For this review, take the finished solid that the model builds, in its own axes (mm). A direction names the side the tool comes from. Give positions to 0.01 mm unless a question says otherwise; leave off trailing zeros. Loops run counter-clockwise (first coordinate to the right, second up) from the corner with the lowest first, then second, coordinate; pieces in that order, holes last. Notation, with made-up numbers: (3, 60.5) - (15, 60.5) arc R26 ccw to (15, 99.5) - close; hole circle Ø3 at (69, 64.25). An arc over 180 degrees is marked (long way). Put each result on its own line as item: value. Start each with the question number.
from build123d import *

# Parameters (mm, degrees)
SKETCH1_W           = 30
SKETCH1_H           = 16
BOSS_EXTRUDE1_DEPTH = 20
CUT_EXTRUDE1_DEPTH  = 20
SKETCH3_W           = 6
SKETCH3_H           = 10
BOSS_EXTRUDE2_DEPTH = 5
SKETCH9_R           = 1.6
CUT_EXTRUDE3_DEPTH  = 6.5
SKETCH11_W          = 10
SKETCH11_H          = 8
BOSS_EXTRUDE4_DEPTH = 40
CHAMFER2_SIZE2      = 10
CHAMFER2_SIZE       = 2
FILLET1_R           = 1
CUT_EXTRUDE4_DEPTH  = 8
SKETCH13_W          = 2
SKETCH13_H          = 8
BOSS_EXTRUDE5_DEPTH = 10
LPATTERN1_COUNT     = 8
LPATTERN1_PITCH     = 5.75
FILLET2_R           = 1
FILLET3_R           = 1
SKETCH14_W          = 2
SKETCH14_H          = 8
CUT_EXTRUDE5_DEPTH  = 5


# Some blends are built 0.0001 mm under size
with BuildPart() as part:
    # Sketch1 → Boss-Extrude1 (new body)
    with BuildSketch(Plane.XY):
        with Locations((15, -8)):
            Rectangle(SKETCH1_W, SKETCH1_H)
    extrude(amount=BOSS_EXTRUDE1_DEPTH)

    # Sketch2 → Cut-Extrude1 (cut)
    with BuildSketch(Plane.XY.offset(20)):
        Polygon((22, -6.5), (22, -8), (30, -8), (30, -16), (6, -16), (6, -6.5), align=None)
    extrude(amount=-CUT_EXTRUDE1_DEPTH, mode=Mode.SUBTRACT)

    # Sketch3 → Boss-Extrude2 (add)
    with BuildSketch(Plane.XZ.offset(16)):
        with Locations((3, 10)):
            Rectangle(SKETCH3_W, SKETCH3_H)
    extrude(amount=BOSS_EXTRUDE2_DEPTH)

    # Sketch9 → Cut-Extrude3 (cut)
    with BuildSketch(Plane.XZ.offset(6.5)):
        with Locations(Location((18, 15, 0), (0, 0, 270))):
            Circle(SKETCH9_R)
        with Locations(Location((18, 5, 0), (0, 0, 270))):
            Circle(SKETCH9_R)
    extrude(amount=-CUT_EXTRUDE3_DEPTH, mode=Mode.SUBTRACT)

    # Sketch11 → Boss-Extrude4 (add)
    with BuildSketch(Plane.XY.offset(15)):
        with Locations((3, -17)):
            Rectangle(SKETCH11_W, SKETCH11_H)
    extrude(amount=BOSS_EXTRUDE4_DEPTH)

    # Chamfer2
    chamfer2_edges = [part.edges().sort_by_distance(p)[0] for p in [
        (0, -17, 15),
    ]]
    chamfer2_side = [part.faces().sort_by_distance(p)[0] for p in [
        (-0.04, -17, 15),
    ]]
    chamfer(chamfer2_edges, length=CHAMFER2_SIZE - 0.0001, length2=CHAMFER2_SIZE2 - 0.0001, reference=chamfer2_side[0])  # a hair under: the kernel refuses the full size

    # Fillet1
    fillet1_edges = [part.edges().sort_by_distance(p)[0] for p in [
        (3, -13, 20),
    ]]
    fillet(fillet1_edges, radius=FILLET1_R)

    # Sketch12 → Cut-Extrude4 (cut)
    with BuildSketch(Plane.XZ.offset(21)):
        Polygon((7, 55), (4.75, 54.25), (2, 53.25), (2, 51.75), (4.75, 50.75), (7, 50), (7, 49.25), (8, 49.25), (8, 55), align=None)
    cut_extrude4 = extrude(amount=-CUT_EXTRUDE4_DEPTH, mode=Mode.SUBTRACT)

    # Sketch13 → Boss-Extrude5 (add)
    with BuildSketch(Plane(origin=(0, 0, 15), x_dir=(-1, 0, 0), z_dir=(0, 0, -1))):
        with Locations((-7, -17)):
            Rectangle(SKETCH13_W, SKETCH13_H)
    extrude(amount=BOSS_EXTRUDE5_DEPTH)

    # LPattern1: Cut-Extrude4 ×8
    with Locations(*[(0, 0, -i * LPATTERN1_PITCH) for i in range(1, LPATTERN1_COUNT)]):
        add(cut_extrude4, mode=Mode.SUBTRACT)

    # Fillet2
    # the kernel refuses this fillet: 1 mm, written as the material it adds along each edge
    with BuildSketch(Plane(origin=(2, -21, 51.75), x_dir=(0.9397934234884382, 0, -0.3417430630867014), z_dir=(0, 1, 0)), Plane(origin=(2, -21, 53.25), x_dir=(0, 0, -1), z_dir=(0, 1, 0)), Plane(origin=(2, -21, 46), x_dir=(0.9397934234884356, 0, -0.34174306308670804), z_dir=(0, 1, 0)), Plane(origin=(2, -21, 47.5), x_dir=(0, 0, -1), z_dir=(0, 1, 0)), Plane(origin=(2, -21, 40.25), x_dir=(0.9397934234884383, 0, -0.3417430630867007), z_dir=(0, 1, 0)), Plane(origin=(2, -21, 41.75), x_dir=(0, 0, -1), z_dir=(0, 1, 0)), Plane(origin=(2, -21, 28.75), x_dir=(0.939793423488437, 0, -0.3417430630867048), z_dir=(0, 1, 0)), Plane(origin=(2, -21, 30.25), x_dir=(0, 0, -1), z_dir=(0, 1, 0)), Plane(origin=(2, -21, 34.5), x_dir=(0.9397934234884383, 0, -0.3417430630867007), z_dir=(0, 1, 0)), Plane(origin=(2, -21, 36), x_dir=(0, 0, -1), z_dir=(0, 1, 0)), Plane(origin=(2, -21, 24.5), x_dir=(0, 0, -1), z_dir=(0, 1, 0)), Plane(origin=(2, -21, 23), x_dir=(0.939793423488437, 0, -0.3417430630867048), z_dir=(0, 1, 0))) as fillet2_piece_1:
        with BuildLine():
            CenterArc((FILLET2_R * 0.700427264611, -FILLET2_R), FILLET2_R, 90, 70.016893478)
            Line((-FILLET2_R * 0.239366158878, -FILLET2_R * 0.658256936913), (0, 0))
            Line((0, 0), (FILLET2_R * 0.700427264611, 0))
        make_face()
    extrude(amount=8)
    with BuildSketch(Plane(origin=(2, -21, 11.5), x_dir=(0.939793423488437, 0, -0.3417430630867044), z_dir=(0, 1, 0)), Plane(origin=(2, -21, 13), x_dir=(0, 0, -1), z_dir=(0, 1, 0)), Plane(origin=(2, -21, 17.25), x_dir=(0.939793423488437, 0, -0.3417430630867048), z_dir=(0, 1, 0))) as fillet2_piece_2:
        with BuildLine():
            CenterArc((FILLET2_R * 0.700427264611, -FILLET2_R), FILLET2_R, 90, 70.016893478)
            Line((-FILLET2_R * 0.239366158878, -FILLET2_R * 0.658256936913), (0, 0))
            Line((0, 0), (FILLET2_R * 0.700427264611, 0))
        make_face()
    extrude(amount=9.751068162)
    with BuildSketch(Plane(origin=(2, -21, 18.75), x_dir=(0.9397934234884369, 0, 0.34174306308670505), z_dir=(0, 1, 0))) as fillet2_piece_3:
        with BuildLine():
            CenterArc((FILLET2_R * 0.700427264611, FILLET2_R), FILLET2_R, 199.983106522, 70.016893478)
            Line((-FILLET2_R * 0.239366158878, FILLET2_R * 0.658256936913), (0, 0))
            Line((0, 0), (FILLET2_R * 0.700427264611, 0))
        make_face()
    extrude(amount=9.751068162)
    # the kernel refuses this fillet: 1 mm, written as the material it takes off along each edge
    with BuildSketch(Plane(origin=(7, -22.80189805, 26.25), x_dir=(-0.9486832980505139, 0, -0.31622776601683794), z_dir=(0, 1, 0)), Plane(origin=(7, -22.80189805, 27), x_dir=(0, 0, -1), z_dir=(0, 1, 0)), Plane(origin=(7, -22.80189805, 32), x_dir=(-0.9486832980505122, 0, -0.31622776601684277), z_dir=(0, 1, 0)), Plane(origin=(7, -22.80189805, 32.75), x_dir=(0, 0, -1), z_dir=(0, 1, 0)), Plane(origin=(7, -22.80189805, 37.75), x_dir=(-0.9486832980505133, 0, -0.31622776601683944), z_dir=(0, 1, 0)), Plane(origin=(7, -22.80189805, 38.5), x_dir=(0, 0, -1), z_dir=(0, 1, 0)), Plane(origin=(7, -22.80189805, 43.5), x_dir=(-0.9486832980505137, 0, -0.31622776601683833), z_dir=(0, 1, 0)), Plane(origin=(7, -22.80189805, 44.25), x_dir=(0, 0, -1), z_dir=(0, 1, 0)), Plane(origin=(7, -22.80189805, 49.25), x_dir=(-0.9486832980505137, 0, -0.31622776601683833), z_dir=(0, 1, 0)), Plane(origin=(7, -22.80189805, 50), x_dir=(0, 0, -1), z_dir=(0, 1, 0)), Plane(origin=(7, -22.80189805, 14.75), x_dir=(-0.9486832980505139, 0, -0.31622776601683794), z_dir=(0, 1, 0)), Plane(origin=(7, -22.80189805, 15.5), x_dir=(0, 0, -1), z_dir=(0, 1, 0)), Plane(origin=(7, -22.80189805, 20.5), x_dir=(-0.9486832980505137, 0, -0.3162277660168387), z_dir=(0, 1, 0)), Plane(origin=(7, -22.80189805, 21.25), x_dir=(0, 0, -1), z_dir=(0, 1, 0))) as fillet2_2_piece_1:
        with BuildLine():
            CenterArc((FILLET2_R * 0.720759220056, FILLET2_R), FILLET2_R, 198.434948823, 71.565051177)
            Line((-FILLET2_R * 0.227924077994, FILLET2_R * 0.683772233983), (0, 0))
            Line((0, 0), (FILLET2_R * 0.720759220056, 0))
        make_face()
    extrude(amount=11.6037961, mode=Mode.SUBTRACT)

    # Fillet3
    # the kernel refuses this fillet: 1 mm, written as the material it takes off along each edge
    with BuildSketch(Plane(origin=(7, -29.045614591, 55), x_dir=(-1, 0, 0), z_dir=(0, 1, 0))) as fillet3_piece_1:
        with BuildLine():
            CenterArc((3.218245837, -1), FILLET3_R, 90, 75.522487814)
            Line((2.25, -0.75), (2.230635083, -0.745))
            ThreePointArc((2.230635083, -0.745), (1.118675445, -0.393973666), (-0.006324555, -0.018973666))
            Line((-0.006324555, -0.018973666), (0, 0.02))
            Line((0, 0.02), (3.218245837, 0.02))
            Line((3.218245837, 0.02), (3.218245837, 0))
        make_face()
    extrude(amount=24.091229183, mode=Mode.SUBTRACT)

    # Sketch14 → Cut-Extrude5 (cut)
    with BuildSketch(Plane(origin=(0, 0, 5), x_dir=(-1, 0, 0), z_dir=(0, 0, -1))):
        with Locations((-7, -17)):
            Rectangle(SKETCH14_W, SKETCH14_H)
    extrude(amount=-CUT_EXTRUDE5_DEPTH, mode=Mode.SUBTRACT)


solid = part.part
1) Take a section at A-A on x = 18. State the section outline as (y, z) points.
2) Mouldability with a two-part tool opening along Z and no side actions: class faces 1 (the flat face through (5.5, -17.1, 50.5)), 2 (the flat face through (5.5, -17.1, 16)), 3 (the flat face through (14, -6.5, 10)) as released by +Z, released by -Z, zero draft, split by the parting line, or undercut.
3) Insertion check: P1, Ø0.8, axis at y = -7.5, z = 15, coming from the -X side; P2, Ø1, axis at x = 6, y = -9.5, coming from the +Z side; P3, Ø2.5, axis at x = 18, z = 5, coming from the -Y side; P4, Ø2.5, axis at x = 26.5, z = 14.5, coming from the -Y side. Each pin has a flat end and moves straight along its axis. Give the tip position at first contact, or say it passes through.
4) Take a section at C-C on z = 4. State the section outline as (x, y) points, and give its area (3 significant figures).
5) Take a section at B-B on y = -5. State the section outline as (x, z) points.
6) Wall thickness on probe 1 along X at (y, z) = (-5, 5); probe 2 along Z at (x, y) = (11, -0.75); probe 3 along X at (y, z) = (-9.5, 17.5): over which ranges is each line inside the solid? List them lowest first.
7) Machinability: for faces 4 (the flat face through (5.522, -17.056, 44.743)), 5 (the flat face through (22, -7, 10)), 6 (the flat face through (3, -18, 5)), 7 (the flat face through (3.719, -17.056, 13.625)), 8 (the flat face through (-2, -17, 35)), which of the approach directions +Z, -Z, +X, -X, +Y, -Y give a long, thin tool a straight path to every point of the face, cutting with its end or side? Answer none if there is none.
8) Take a section at D-D on y = -9.25. State the section outline as (x, z) points, and give its area (3 significant figures).
Answers follow:
1. outline: (-6.5, 0) - (0, 0) - (0, 3.4) - (-6.5, 3.4) - close; (-6.5, 6.6) - (0, 6.6) - (0, 13.4) - (-6.5, 13.4) - close; (-6.5, 16.6) - (0, 16.6) - (0, 20) - (-6.5, 20) - close
2. face 1: released by +Z
2. face 2: undercut
2. face 3: zero draft
3. P1: x = 0
3. P2: z = 20
3. P3: through
3. P4: y = -8
4. outline: (0, -16) - (6, -16) - (6, -6.5) - (16.75, -6.5) - (16.75, 0) - (0, 0) - close; (19.25, -6.5) - (22, -6.5) - (22, -8) - (30, -8) - (30, 0) - (19.25, 0) - close
4. area: 248 mm2
5. outline: (0, 0) - (30, 0) - (30, 20) - (0, 20) - close; hole circle Ø3.2 at (18, 5); hole circle Ø3.2 at (18, 15)
6. probe 1: 0 to 16.4, 19.6 to 30
6. probe 2: 0 to 20
6. probe 3: 0 to 6
7. face 4: +X, +Y, -Y
7. face 5: +Z, -Z, -Y
7. face 6: -Z, +X, -X, -Y
7. face 7: +X, -Y
7. face 8: +Z, -Z, -X, +Y, -Y
8. outline: (0, 0) - (6, 0) - (6, 20) - (0, 20) - close
8. area: 120 mm2
